from build123d import *

# Parameters (mm, degrees)
F0_R     = 38.1
F1_DEPTH = 31.75
F2_R     = 12.7
F3_DEPTH = 152.4
F4_W     = 38.1
F4_H     = 101.6
F4_W_2   = 75.343641
F5_DEPTH = 63.5
F7_DEPTH = 152.401


with BuildPart() as f1:
    # F0 (on Front) → F1 (new body)
    with BuildSketch(Plane.XZ):
        with BuildLine():
            ThreePointArc((0, -76.2), (53.881537, -53.881537), (76.2, 0))
            ThreePointArc((76.2, 0), (53.881537, 53.881537), (0, 76.2))
            ThreePointArc((0, 76.2), (-76.2, 0), (0, -76.2))
        make_face()
        Circle(F0_R, mode=Mode.SUBTRACT)
        with BuildLine():
            ThreePointArc((0, 76.2), (53.881537, 53.881537), (76.2, 0))
            ThreePointArc((76.2, 0), (53.881537, -53.881537), (0, -76.2))
            Line((0, -76.2), (101.6, -76.2))
            Line((101.6, -76.2), (101.6, 76.2))
            Line((101.6, 76.2), (0, 76.2))
        make_face()
    extrude(amount=F1_DEPTH)

    # F2 (on face) → F3 (join)
    with BuildSketch(Plane.XY.offset(76.2)):
        with BuildLine():
            Line((101.6, 0), (101.6, -31.75))
            ThreePointArc((101.6, -31.75), (146.827869, -15.875), (101.6, 0))
        make_face()
        with Locations((121.427869, -15.875)):
            Circle(F2_R, mode=Mode.SUBTRACT)
    extrude(amount=-F3_DEPTH)

    # F4 (on face) → F5 (cut, symmetric)
    with BuildSketch(Plane.XZ.offset(31.75)):
        with Locations((107.95, 0)):
            Rectangle(F4_W, F4_H)
        with Locations((164.67182, 0)):
            Rectangle(F4_W_2, F4_H)
    extrude(amount=F5_DEPTH, both=True, mode=Mode.SUBTRACT)

    # F6 (on face) → F7 (cut, through all)
    with BuildSketch(Plane.XY.offset(76.2)):
        with BuildLine():
            Line((7.127869, -19.05), (57.927869, -19.05))
            ThreePointArc((57.927869, -19.05), (61.102869, -15.875), (57.927869, -12.7))
            Line((57.927869, -12.7), (7.127869, -12.7))
            ThreePointArc((7.127869, -12.7), (3.952869, -15.875), (7.127869, -19.05))
        make_face()
    extrude(amount=-F7_DEPTH, mode=Mode.SUBTRACT)


solid = f1.part
Here's how the part is built. I have some questions about the finished solid (model axes, mm). A direction names the side the tool comes from. Give positions to 0.01 mm unless a question says otherwise; leave off trailing zeros. Loops run counter-clockwise (first coordinate to the right, second up) from the corner with the lowest first, then second, coordinate; pieces in that order, holes last. Notation, with made-up numbers: (3, 19.25) -> (51, 19.25) arc R25 cw to (51, 42.25) -> close; hole circle Ø6 at (24.25, 42.25). An arc over 180 degrees is marked (long way). One line per item, written item: value.
Q1. Suppose I cut it at D-D on z = 42. Please give me the cut outline in (x, y) (3 decimals), then the cut area to 3 significant figures.
Answers follow:
outline: (-63.58, -31.75) -> (88.9, -31.75) -> (88.9, 0) -> (-63.58, 0) -> close; hole (7.128, -19.05) -> (57.928, -19.05) arc R3.175 ccw to (57.928, -12.7) -> (7.128, -12.7) arc R3.175 ccw to start
area: 4,490 mm^2
Q2. Suppose I cut it at C-C on y = -22. Please give me the cut outline in (x, z), then the cut area to 3 significant figures.
Answers follow:
outline: (0, -76.2) -> (110.3, -76.2) -> (110.3, -50.8) -> (88.9, -50.8) -> (88.9, 50.8) -> (110.3, 50.8) -> (110.3, 76.2) -> (0, 76.2) arc R76.2 ccw to start; (132.55, -76.2) -> (146.08, -76.2) -> (146.08, -50.8) -> (132.55, -50.8) -> close; (132.55, 50.8) -> (146.08, 50.8) -> (146.08, 76.2) -> (132.55, 76.2) -> close; hole circle Ø76.2 at (0, 0)
area: 19,900 mm^2
Q3. If I drill on line 1 along Y through (x, z) = (55, -21); line 2 along Z through (x, y) = (119, -29.5); line 3 along Y through (x, z) = (76.5, 19), over which ranges is the centre line in solid material (lowest first)?
Answers follow:
line 1: -31.75 to -19.05, -12.7 to 0
line 2: -76.2 to -50.8, 50.8 to 76.2
line 3: -31.75 to 0
Q4. On a 3-axis mill with a long thin cutter (end or side, diameter ignored), from which of +Z, -Z, +X, -X, +Y, -Y can I reach the whole of each face in a straight line? I mean faces 4 (the face through (111, -5, -50.8)), 5 (the face through (31, 0, 35)), 6 (the face through (43, -19.05, 1)), 7 (the face through (31, -31.75, 35)). Say none if no direction works.
Answers follow:
face 4: +X, +Y, -Y
face 5: +Z, -Z, -X, +Y
face 6: +Z, -Z
face 7: +Z, -Z, -X, -Y
Q5. I'm going to push flat-ended pins straight in: pin 1 Ø23 at (x, y) = (121.43, -15.88) entering from -Z; pin 2 Ø2 at (y, z) = (-21.5, -45) entering from -X; pin 3 Ø12 at (y, z) = (-30, 8) entering from +X; pin 4 Ø1 at (x, z) = (-26.5, -43) entering from -Y. Where does each tip first touch, or does it pass through?
Answers follow:
pin 1: through
pin 2: x = -62.21
pin 3: x = 88.9
pin 4: y = -31.75
Q6. Suppose I cut it at A-A on x = 44. Please give me the cut outline in (y, z).
Answers follow:
outline: (-31.75, -76.2) -> (-19.05, -76.2) -> (-19.05, 76.2) -> (-31.75, 76.2) -> close; (-12.7, -76.2) -> (0, -76.2) -> (0, 76.2) -> (-12.7, 76.2) -> close
Q7. Suppose I cut it at B-B on z = 0. Please give me the cut outline in (x, y) (3 decimals).
Answers follow:
outline: (-76.2, -31.75) -> (-38.1, -31.75) -> (-38.1, 0) -> (-76.2, 0) -> close; (38.1, -31.75) -> (88.9, -31.75) -> (88.9, 0) -> (38.1, 0) -> (38.1, -12.7) -> (57.928, -12.7) arc R3.175 cw to (57.928, -19.05) -> (38.1, -19.05) -> close
Q8. We'd pull the mould along Z, two halves only. Please class faces 1 (the face through (3.954, -15.805, 57.085)), 2 (the face through (72, -16, -76.2)), 3 (the face through (88.9, -16, -1)): pulls with the +Z half, pulls with the -Z half, needs draft (parallel to the pull), parting line crosses it, or undercut.
Answers follow:
face 1: needs draft
face 2: pulls with the -Z half
face 3: undercut
